```python
from build123d import *

# Parameters (mm, degrees)
SKETCH1_R           = 10
BOSS_EXTRUDE1_DEPTH = 20
SKETCH2_W           = 10
SKETCH2_H           = 35
CUT_EXTRUDE1_DEPTH  = 20


with BuildPart() as part:
    # Sketch1 → Boss-Extrude1 (new body)
    with BuildSketch(Plane.XY):
        with BuildLine():
            Line((-4.771193235, -41.306779105), (0.228806765, -41.306779105))
            Line((0.228806765, -41.306779105), (0.228806765, -86.306779105))
            Line((0.228806765, -86.306779105), (10.228806765, -86.306779105))
            Line((10.228806765, -86.306779105), (10.228806765, -41.306779105))
            Line((10.228806765, -41.306779105), (15.228806765, -41.306779105))
            ThreePointArc((15.228806765, -41.306779105), (20.581175565, -25.848105545), (34.346453824, -17.008673749))
            ThreePointArc((34.346453824, -17.008673749), (46.902822198, 5.31292851), (23.747325283, 16.255472857))
            ThreePointArc((23.747325283, 16.255472857), (5.228806765, 12.69968102), (-13.289711754, 16.255472857))
            ThreePointArc((-13.289711754, 16.255472857), (-36.445208668, 5.31292851), (-23.888840294, -17.008673749))
            ThreePointArc((-23.888840294, -17.008673749), (-10.123562035, -25.848105545), (-4.771193235, -41.306779105))
        make_face()
        with Locations((-19.771193235, 0)):
            Circle(SKETCH1_R, mode=Mode.SUBTRACT)
        with Locations((30.228806765, 0)):
            Circle(SKETCH1_R, mode=Mode.SUBTRACT)
    extrude(amount=BOSS_EXTRUDE1_DEPTH)

    # Sketch2 → Cut-Extrude1 (cut)
    with BuildSketch(Plane(origin=(10.228806765, 0, 0), x_dir=(0, 0, -1), z_dir=(1, 0, 0))):
        with Locations((-10, -68.806779105)):
            Rectangle(SKETCH2_W, SKETCH2_H)
    extrude(amount=-CUT_EXTRUDE1_DEPTH, mode=Mode.SUBTRACT)


solid = part.part
```
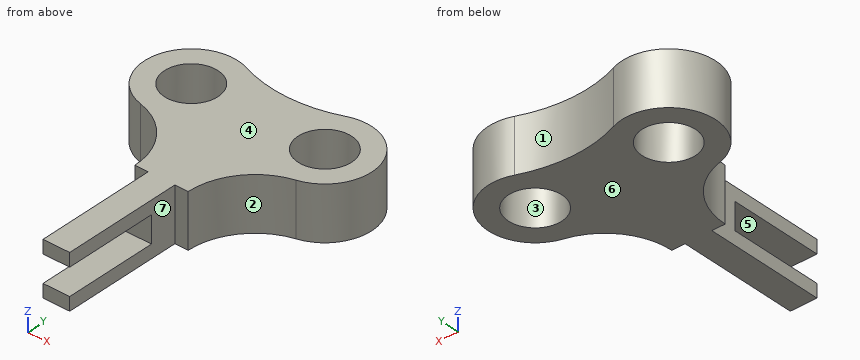
The model under review builds one solid part; all positions refer to its coordinate system, in mm. Face numbers are marked on the shaded views. A direction names the side the tool comes from. Round coordinates to 2 decimals unless told otherwise and drop trailing zeros. Order: outer loops, then holes, each group sorted by start corner. A loop starts at its lowest first (then second) coordinate and runs counter-clockwise, first axis right, second up.
(1) Take a section at C-C, the plane x = 33. State the section outline as (y, z) points, plus the area to 3 significant figures.
Working result:
outline: (-17.37, 0) - (-9.61, 0) - (-9.61, 20) - (-17.37, 20) - close; (9.61, 0) - (17.28, 0) - (17.28, 20) - (9.61, 20) - close
area: 309 mm2
(2) Take a section at A-A, the plane z = 11.5. State the section outline as (x, y) points, plus the area to 3 significant figures.
Working result:
outline: (-23.89, -17.01) arc R25 cw to (-4.77, -41.31) - (0.23, -41.31) - (0.23, -51.31) - (10.23, -51.31) - (10.23, -41.31) - (15.23, -41.31) arc R25 cw to (34.35, -17.01) arc R17.5 ccw (long way) to (23.75, 16.26) arc R50 cw to (-13.29, 16.26) arc R17.5 ccw (long way) to start; hole circle Ø20 at (-19.77, 0); hole circle Ø20 at (30.23, 0)
area: 2,740 mm2
(3) Wall thickness on L1, parallel to X at y = -6.5, z = 14.5; L2, parallel to Y at x = -28.5, z = 4.25; L3, parallel to Y at x = 5.5, z = 8.5: over which ranges is each line inside the solid? List them lowest first.
Working result:
L1: x = -36.02 to -27.37, -12.17 to 22.63, 37.83 to 46.48
L2: y = -15.17 to -4.88, 4.88 to 15.17
L3: y = -51.31 to 12.7
(4) Take a section at D-D, the plane y = 0. State the section outline as (x, z) points.
Working result:
outline: (-37.27, 0) - (-29.77, 0) - (-29.77, 20) - (-37.27, 20) - close; (-9.77, 0) - (20.23, 0) - (20.23, 20) - (-9.77, 20) - close; (40.23, 0) - (47.73, 0) - (47.73, 20) - (40.23, 20) - close
(5) Take a section at B-B, the plane y = -72. State the section outline as (x, z) points.
Working result:
outline: (0.23, 0) - (10.23, 0) - (10.23, 5) - (0.23, 5) - close; (0.23, 15) - (10.23, 15) - (10.23, 20) - (0.23, 20) - close
(6) Tool access review of the marked faces 5, 6 and 7: name each direction out of +Z, -Z, +X, -X, +Y, -Y from which nothing blocks a thin tool from reaching the whole face with its end or side.
Working result:
face 5: +X, -X, -Y
face 6: -Z, +X, -X, +Y, -Y
face 7: +Z, -Z, +X, -Y
(7) For P1, Ø12, axis at x = -27.5, y = -23, coming from the -Z side; P2, Ø1.5, axis at x = -0.5, z = 6.5, coming from the +Y side; P3, Ø10, axis at y = -26.5, z = 3, coming from the +X side; P4, Ø10, axis at y = -61.5, z = 8.5, coming from the -X side, all flat-tipped, find the tip position at first contact; note any pin that passes through.
Working result:
P1: passes through
P2: stops at y = 13.12
P3: stops at x = 24.97
P4: stops at x = 0.23
(8) Mouldability with a two-part tool opening along X and no side actions: class the marked faces 1, 2, 3 and 4 as released by +X, released by -X, zero draft, split by the parting line, or undercut.
Working result:
face 1: undercut
face 2: released by +X
face 3: undercut
face 4: zero draft
